Work out the finished part from the listing and answer in its coordinate system (mm). A direction names the side the tool comes from. Coordinates: 2 decimals unless noted, no trailing zeros. Order: outer loops, then holes, each group sorted by start corner. A loop starts at its lowest first (then second) coordinate and runs counter-clockwise, first axis right, second up. Notation, with made-up numbers: M 48.5,77.5 L 80.5,77.5 A35 ccw 80.5,114.5 Z; hole C 82,-25 d11. An arc over 180 degrees is marked long. Write item = value, one per line. Start each with the question number.
Q1. Find section A-A on x = -12.5. Give the vertices of the cut face in (y, z).
Q2. Each of these flat-tipped pins is pushed along its axis until it touches: P1, Ø8, axis at x = -5.5, y = 2.5, coming from the -Z side; P2, Ø2, axis at y = 7.5, z = 11.5, coming from the +X side; P3, Ø0.6, axis at x = -11, z = 10.5, coming from the -Y side; P4, Ø4, axis at x = 10.09, y = 4.75, coming from the +Z side. Where does it stop, or does it pass through?
Q3. Find section C-C on z = 9. Give the vertices of the cut face in (x, y).
Q4. Determine the mould class of faces 1 (the flat face through (-8.5, 7, 11)), 2 (the flat face through (-6, -10, 6)), 3 (the flat face through (-13, 8, 11)), 4 (the flat face through (-13, -6, 11)) for opening direction Y: released by +Y, released by -Y, zero draft, split by the parting line, or undercut.
Q5. Find section D-D on z = 2.25. Give the vertices of the cut face in (x, y).
Q6. Straight lines are drawn through the part: line 1 along X through (y, z) = (4.75, 7.05); line 2 along Y through (x, z) = (19.59, 7); line 3 along Y through (x, z) = (-12.5, 7.75). For each, find the intervals that lie inside material, in ascending order.
Q7. A tool of negligible diameter and unlimited length cuts with its end or side. For faces 5 (the flat face through (-16.5, -7, 11)), 6 (the flat face through (-13, 6, 11)), 7 (the flat face through (-13, -4, 4)), 8 (the flat face through (-13, -8, 11)), from which of +Z, -Z, +X, -X, +Y, -Y can it reach the whole face along a straight path? Write none if from no direction.
Q8. Find section B-B on y = 0. Give the vertices of the cut face in (x, z).
```python
from build123d import *

# Parameters (mm, degrees)
F0_W     = 55
F0_H     = 20
F0_R     = 3.5
F0_R_2   = 1.5
F1_DEPTH = 10
F2_W     = 8
F2_H     = 2
F3_DEPTH = 2
F4_R     = 5.5
F5_DEPTH = 4
F6_W     = 25
F6_H     = 20
F7_DEPTH = 6


with BuildPart() as f1:
    # F0 (on Top) → F1 (new body)
    with BuildSketch(Plane.XY):
        Rectangle(F0_W, F0_H)
        with Locations((-12.5, 0)):
            Circle(F0_R, mode=Mode.SUBTRACT)
        with Locations((10.09, 4.75)):
            Circle(F0_R_2, mode=Mode.SUBTRACT)
        with Locations((19.59, 4.75)):
            Circle(F0_R_2, mode=Mode.SUBTRACT)
    extrude(amount=F1_DEPTH)

    # F2 (on face) → F3 (join)
    with BuildSketch(Plane.XY.offset(10)):
        with Locations((-12.5, 7)):
            Rectangle(F2_W, F2_H)
        with Locations((-12.5, -7)):
            Rectangle(F2_W, F2_H)
    extrude(amount=F3_DEPTH)

    # F4 (on Top) → F5 (cut)
    with BuildSketch(Plane.XY):
        with Locations((-12.5, 0)):
            Circle(F4_R)
    extrude(amount=F5_DEPTH, mode=Mode.SUBTRACT)

    # F6 (on Top) → F7 (cut)
    with BuildSketch(Plane.XY):
        with Locations((15, 0)):
            Rectangle(F6_W, F6_H)
    extrude(amount=F7_DEPTH, mode=Mode.SUBTRACT)


solid = f1.part
```
Findings below:
q1.outline = M -10,0 L -5.5,0 L -5.5,4 L -3.5,4 L -3.5,10 L -6,10 L -6,12 L -8,12 L -8,10 L -10,10 Z; M 3.5,4 L 5.5,4 L 5.5,0 L 10,0 L 10,10 L 8,10 L 8,12 L 6,12 L 6,10 L 3.5,10 Z
q2.P1 = 0
q2.P2 = -8.5
q2.P3 = -8
q2.P4 = 10
q3.outline = M -27.5,-10 L 27.5,-10 L 27.5,10 L -27.5,10 Z; hole C -12.5,0 d7; hole C 10.09,4.75 d3; hole C 19.59,4.75 d3
q4.face_1 = zero draft
q4.face_2 = released by -Y
q4.face_3 = released by +Y
q4.face_4 = undercut
q5.outline = M -27.5,-10 L 2.5,-10 L 2.5,10 L -27.5,10 Z; hole C -12.5,0 d11
q6.line_1 = -27.5 to 8.59, 11.59 to 18.09, 21.09 to 27.5
q6.line_2 = -10 to 3.25, 6.25 to 10
q6.line_3 = -10 to -3.5, 3.5 to 10
q7.face_5 = +Z, -X, +Y, -Y
q7.face_6 = +Z, +X, -X
q7.face_7 = -Z
q7.face_8 = +Z, +X, -X, -Y
q8.outline = M -27.5,0 L -18,0 L -18,4 L -16,4 L -16,10 L -27.5,10 Z; M -9,4 L -7,4 L -7,0 L 2.5,0 L 2.5,6 L 27.5,6 L 27.5,10 L -9,10 Z
